from build123d import *

# Parameters (mm, degrees)
SCHIZZO1_W                   = 15
SCHIZZO1_H                   = 24.2
SCHIZZO1_R                   = 4.25
ESTRUSIONE_ESTRUSIONE1_DEPTH = 7.5
TAGLIO_ESTRUSIONE1_REACH     = 22.68


with BuildPart() as part:
    # Schizzo1 → Estrusione-Estrusione1 (new, symmetric)
    with BuildSketch(Plane.XY):
        Rectangle(SCHIZZO1_W, SCHIZZO1_H)
        with Locations((0, -4.6)):
            Circle(SCHIZZO1_R, mode=Mode.SUBTRACT)
    extrude(amount=ESTRUSIONE_ESTRUSIONE1_DEPTH, both=True)

    # Schizzo2 → Taglio-Estrusione1 (cut, up to next)
    with BuildSketch(Plane.ZY.offset(7.5), mode=Mode.PRIVATE) as taglio_estrusione1_sk1:
        with BuildLine():
            Line((4.25, 2.146261356), (4.25, 7.053738644))
            Line((4.25, 7.053738644), (2.125, 8.280607966))
            ThreePointArc((2.125, 8.280607966), (-4.25, 4.6), (2.125, 0.919392034))
            Line((2.125, 0.919392034), (4.25, 2.146261356))
        make_face()
    taglio_estrusione1_tool1 = extrude(taglio_estrusione1_sk1.sketch, amount=-TAGLIO_ESTRUSIONE1_REACH, mode=Mode.PRIVATE) & part.part
    add(taglio_estrusione1_tool1.solids().sort_by_distance((-7.5, 4.6, 0.125868))[0], mode=Mode.SUBTRACT)


solid = part.part
Could you check a few things on this model? Use its own coordinates, in mm. A direction names the side the tool comes from. Coordinates: 2 decimals unless noted, no trailing zeros. Order: outer loops, then holes, each group sorted by start corner. A loop starts at its lowest first (then second) coordinate and runs counter-clockwise, first axis right, second up.
Q1. Which directions (+Z, -Z, +X, -X, +Y, -Y) give clear straight access to the entire face, cutting with the end or side of a thin tool? Please do faces 4 (the flat face through (0, 12.1, 0)), 5 (the flat face through (-0.105, 1.524, 3.173)).
Q2. Suppose I cut it at D-D on x = 3.75. Please give me the cut outline in (y, z) (3 decimals).
Q3. Thinking about a two-plate mould opening in Z: for faces 1 (the flat face through (7.5, 0, 0)), 2 (the flat face through (-0.11, 7.66, 3.2)), 3 (the flat face through (0, 0, 7.5)), which applies, released by +Z, released by -Z, zero draft, split by the parting line, or undercut?
Q4. Will this pin go through, and if not, where does the flat tip stop? pin 1 (2 mm diameter, centred on x = -3, y = -3.5, fed in from -Z).
Q5. Suppose I cut it at B-B on y = 4.6. Please give me the cut outline in (x, z).
Q6. Suppose I cut it at A-A on x = 0. Please give me the cut outline in (y, z) (3 decimals).
Q7. Suppose I cut it at C-C on z = 0. Please give me the cut outline in (x, y).
Q8. Please list where these lines run through material, in increasing order: L1, parallel to Y at x = 0.5, z = 0; L2, parallel to Y at x = -2, z = 7.25; L3, parallel to Y at x = 1.75, z = 1.25.
Answer:
1. face 4: +Z, -Z, +X, -X, +Y
1. face 5: +X, -X
2. outline: (-12.1, -7.5) - (-6.6, -7.5) - (-6.6, 7.5) - (-12.1, 7.5) - close; (-2.6, -7.5) - (12.1, -7.5) - (12.1, 7.5) - (-2.6, 7.5) - close; hole (0.919, 2.125) arc R4.25 ccw (long way) to (8.281, 2.125) - (7.054, 4.25) - (2.146, 4.25) - close
3. face 1: zero draft
3. face 2: undercut
3. face 3: released by +Z
4. pin 1: passes through
5. outline: (-7.5, -7.5) - (7.5, -7.5) - (7.5, -4.25) - (-7.5, -4.25) - close; (-7.5, 4.25) - (7.5, 4.25) - (7.5, 7.5) - (-7.5, 7.5) - close
6. outline: (-12.1, -7.5) - (-8.85, -7.5) - (-8.85, 7.5) - (-12.1, 7.5) - close; (-0.35, -7.5) - (12.1, -7.5) - (12.1, 7.5) - (-0.35, 7.5) - close; hole (0.919, 2.125) arc R4.25 ccw (long way) to (8.281, 2.125) - (7.054, 4.25) - (2.146, 4.25) - close
7. outline: (-7.5, -12.1) - (7.5, -12.1) - (7.5, 0.35) - (-7.5, 0.35) - close; (-7.5, 8.85) - (7.5, 8.85) - (7.5, 12.1) - (-7.5, 12.1) - close; hole circle Ø8.5 at (0, -4.6)
8. L1: y = -12.1 to -8.82, -0.38 to 0.35, 8.85 to 12.1
8. L2: y = -12.1 to -8.35, -0.85 to 12.1
8. L3: y = -12.1 to -8.47, -0.73 to 0.54, 8.66 to 12.1
